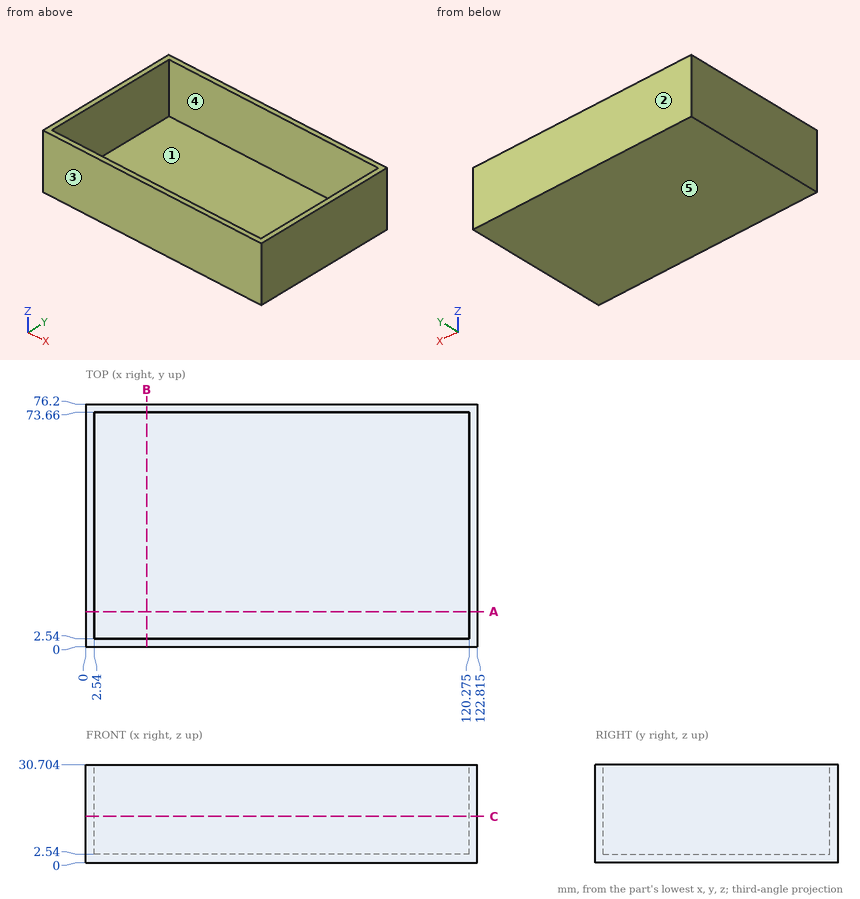
Here's the drawing with two shaded views (mm, measured from the low corner). I have some questions. A direction names the side the tool comes from. Give positions to 0.01 mm unless a question says otherwise; leave off trailing zeros. Loops run counter-clockwise (first coordinate to the right, second up) from the corner with the lowest first, then second, coordinate; pieces in that order, holes last. Notation, with made-up numbers: M -15,37.5 L 43,37.5 A11 ccw 43,47.5 Z; hole C 58.5,27.25 d2. An arc over 180 degrees is marked long. Use one line per item in the form item = value. Start each with the question number.
Q1. If we section it at B-B (x = 19): Write out the boundary of the cut face in (y, z).
Q2. I need wall thicknesses on line 1 along Y through (x, z) = (69, 19); line 2 along X through (y, z) = (9, 23) (1 decimal); line 3 along Z through (x, y) = (106, 47). Which ranges of each line are inside material? Lowest first, please.
Q3. If we section it at A-A (y = 11): Write out the boundary of the cut face in (x, z) (1 decimal), then the cut area to 3 significant figures.
Q4. Thinking about a two-plate mould opening in Y: for the marked faces 1, 2 and 3, which applies, +Y half, -Y half, draft (parallel to the pull), parting line (faces both ways), or undercut?
Q5. Which directions (+Z, -Z, +X, -X, +Y, -Y) give clear straight access to the entire face, cutting with the end or side of a thin tool? Please do the marked faces 4 and 5.
Q6. If we section it at C-C (z = 14.5): Write out the boundary of the cut face in (x, y) (1 decimal).
Q7. Will this pin go through, and if not, where does the flat tip stop? pin 1 Ø8 at (y, z) = (65, 22) entering from -X.
Taken from the geometry:
q1.outline = M 0,0 L 76.2,0 L 76.2,30.7 L 73.66,30.7 L 73.66,2.54 L 2.54,2.54 L 2.54,30.7 L 0,30.7 Z
q2.line_1 = 0 to 2.54, 73.66 to 76.2
q2.line_2 = 0 to 2.5, 120.3 to 122.8
q2.line_3 = 0 to 2.54
q3.outline = M 0,0 L 122.8,0 L 122.8,30.7 L 120.3,30.7 L 120.3,2.5 L 2.5,2.5 L 2.5,30.7 L 0,30.7 Z
q3.area = 455 mm^2
q4.face_1 = undercut
q4.face_2 = +Y half
q4.face_3 = -Y half
q5.face_4 = +Z
q5.face_5 = -Z, +X, -X, +Y, -Y
q6.outline = M 0,0 L 122.8,0 L 122.8,76.2 L 0,76.2 Z; hole M 2.5,2.5 L 120.3,2.5 L 120.3,73.7 L 2.5,73.7 Z
q7.pin_1 = 0
